Answer from the drawing. Dimensions are ordinates in mm from the lowest x, y and z of the part. A direction names the side the tool comes from. Round coordinates to 2 decimals unless told otherwise and drop trailing zeros. Order: outer loops, then holes, each group sorted by start corner. A loop starts at its lowest first (then second) coordinate and runs counter-clockwise, first axis right, second up. Notation, with made-up numbers: (73.25, -39) -> (120.25, -39) arc R30 ccw to (120.25, -12) -> close; hole circle Ø4 at (23, 22). An arc over 180 degrees is marked (long way). Use a Markdown table: item, result. Add a question column.
Item 1: A cutting plane is placed at B-B, the plane y = 4. Determine the outline of the cut face in (x, z), plus the area to 3 significant figures.
Item 2: Find the intervals of material crossed by L1, parallel to X at y = 52, z = 70; L2, parallel to X at y = 26, z = 107, in increasing order. Write a range as [from, to].
Item 3: A cutting plane is placed at D-D, the plane x = 124.5. Determine the outline of the cut face in (y, z).
Item 4: Flat-ended cylindrical pins translate along their axes: P1, Ø2, axis at x = 67, z = 99.5, coming from the -Y side; P2, Ø24.5, axis at x = 88.5, z = 83.5, coming from the +Y side; P3, Ø3, axis at x = 3.5, y = 8.5, coming from the +Z side. Find the tip coordinate at first contact, or state that the pin passes through.
Item 5: A cutting plane is placed at C-C, the plane z = 23.5. Determine the outline of the cut face in (x, y).
Item 6: For a pull along X with two mould halves and no side action, classify the marked faces 1, 2 and 3 as +X half, -X half, draft (parallel to the pull), parting line (faces both ways), or undercut.
Item 7: A tool of negligible diameter and unlimited length cuts with its end or side. For the marked faces 4, 5 and 6, from which of +Z, -Z, +X, -X, +Y, -Y can it reach the whole face along a straight path? Write none if from no direction.
Item 8: A cutting plane is placed at A-A, the plane x = 70. Determine the outline of the cut face in (y, z), plus the area to 3 significant figures.
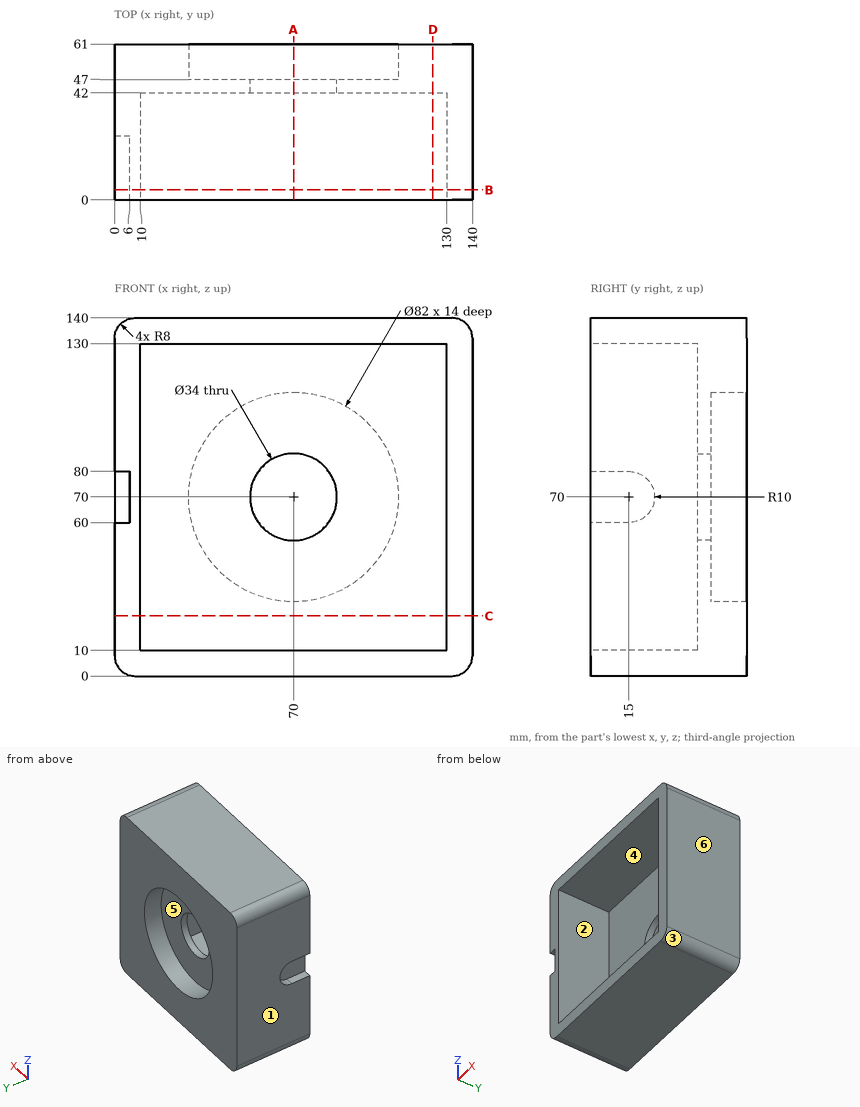
Reported:
| question | item | result |
|---|---|---|
| 1 | outline | (0, 8) arc R8 ccw to (8, 0) -> (132, 0) arc R8 ccw to (140, 8) -> (140, 132) arc R8 ccw to (132, 140) -> (8, 140) arc R8 ccw to (0, 132) -> (0, 80) -> (6, 80) -> (6, 60) -> (0, 60) -> close; hole (10, 10) -> (130, 10) -> (130, 130) -> (10, 130) -> close |
| 1 | area | 5,030 mm² |
| 2 | L1 | [0, 29], [111, 140] |
| 2 | L2 | [0, 10], [130, 140] |
| 3 | outline | (0, 0) -> (61, 0) -> (61, 140) -> (0, 140) -> (0, 130) -> (42, 130) -> (42, 10) -> (0, 10) -> close |
| 4 | P1 | y = 42 |
| 4 | P2 | y = 47 |
| 4 | P3 | z = 139.42 |
| 5 | outline | (0, 0) -> (10, 0) -> (10, 42) -> (130, 42) -> (130, 0) -> (140, 0) -> (140, 61) -> (0, 61) -> close |
| 6 | face 1 | -X half |
| 6 | face 2 | undercut |
| 6 | face 3 | +X half |
| 7 | face 4 | -Y |
| 7 | face 5 | +Y |
| 7 | face 6 | +Z, -Z, +X, +Y, -Y |
| 8 | outline | (0, 0) -> (61, 0) -> (61, 29) -> (47, 29) -> (47, 53) -> (42, 53) -> (42, 10) -> (0, 10) -> close; (0, 130) -> (42, 130) -> (42, 87) -> (47, 87) -> (47, 111) -> (61, 111) -> (61, 140) -> (0, 140) -> close |
| 8 | area | 2,180 mm² |
